Check sheet for the modelled part. Datum: model origin and axes. Units: mm. Round coordinates to 2 decimals unless told otherwise and drop trailing zeros. Order: outer loops, then holes, each group sorted by start corner. A loop starts at its lowest first (then second) coordinate and runs counter-clockwise, first axis right, second up.
Q1. Cross-section at C-C on z = 1.75. Record the cut outline in (x, y).
Q2. Mould release check, pull along X, two halves, no side actions. Record for faces 1 (the flat face through (-31.851, 4, 8)), 2 (the cylindrical face through (28.412, 4.676, 7.736)), 3 (the flat face through (3, 4, 15.341)), 4 (the flat face through (36.149, 4, 8)): +X half, -X half, draft (parallel to the pull), parting line (faces both ways), or undercut.
Q3. Depth check by flat-ended pin: P1, Ø3, axis at x = -13.5, y = 5, coming from the -Z side; P2, Ø1.6, axis at x = 29.15, y = 4, coming from the -Z side. Enter the tip coordinate at first touch or a pass-through.
Q4. Cross-section at A-A on y = 4. Record the cut outline in (x, z), then the cut area to 3 significant figures.
Q5. Cross-section at B-B on x = 29. Record the cut outline in (y, z).
Q6. Scan lines: probe 1 along X at (y, z) = (4, 9.25); probe 2 along Z at (x, y) = (-7, 2); probe 3 along X at (y, z) = (4, 3.75). Record each from-to range of solid material in increasing order.
Q7. Cross-section at D-D on y = 1. Record the cut outline in (x, z), then the cut area to 3 significant figures.
from build123d import *

# Parameters (mm, degrees)
BOSS_EXTRUDE1_DEPTH = 8
SKETCH2_R           = 1
CUT_EXTRUDE1_DEPTH  = 16.340604027


with BuildPart() as part:
    # Sketch1 → Boss-Extrude1 (new body)
    with BuildSketch(Plane(origin=(0, 0, 0), x_dir=(1, 0, 0), z_dir=(0, 1, 0))):
        with BuildLine():
            Line((2.649328859, -0.340604027), (36.149328859, -0.340604027))
            Line((36.149328859, -0.340604027), (36.149328859, -15.340604027))
            Line((36.149328859, -15.340604027), (-31.850671141, -15.340604027))
            Line((-31.850671141, -15.340604027), (-31.850671141, -0.340604027))
            Line((-31.850671141, -0.340604027), (-17.350671141, -0.340604027))
            ThreePointArc((-17.350671141, -0.340604027), (-7.350671141, -10.340604027), (2.649328859, -0.340604027))
        make_face()
    extrude(amount=BOSS_EXTRUDE1_DEPTH)

    # Sketch2 → Cut-Extrude1 (cut, through all)
    with BuildSketch(Plane.XY):
        with Locations((-24.850671141, 4)):
            Circle(SKETCH2_R)
        with Locations((29.149328859, 4)):
            Circle(SKETCH2_R)
    extrude(amount=CUT_EXTRUDE1_DEPTH, mode=Mode.SUBTRACT)


solid = part.part
Results found:
1. outline: (-31.85, 0) - (-17.25, 0) - (-17.25, 8) - (-31.85, 8) - close; (2.55, 0) - (36.15, 0) - (36.15, 8) - (2.55, 8) - close; hole circle Ø2 at (-24.85, 4); hole circle Ø2 at (29.15, 4)
2. face 1: -X half
2. face 2: undercut
2. face 3: draft
2. face 4: +X half
3. P1: stops at z = 6.78
3. P2: passes through
4. outline: (-31.85, 0.34) - (-25.85, 0.34) - (-25.85, 15.34) - (-31.85, 15.34) - close; (-23.85, 0.34) - (-17.35, 0.34) arc R10 cw to (2.65, 0.34) - (28.15, 0.34) - (28.15, 15.34) - (-23.85, 15.34) - close; (30.15, 0.34) - (36.15, 0.34) - (36.15, 15.34) - (30.15, 15.34) - close
4. area: 803 mm2
5. outline: (0, 0.34) - (3.01, 0.34) - (3.01, 15.34) - (0, 15.34) - close; (4.99, 0.34) - (8, 0.34) - (8, 15.34) - (4.99, 15.34) - close
6. probe 1: x = -31.85 to -25.85, -23.85 to -11.89, -2.81 to 28.15, 30.15 to 36.15
6. probe 2: z = 10.33 to 15.34
6. probe 3: x = -31.85 to -25.85, -23.85 to -16.75, 2.05 to 28.15, 30.15 to 36.15
7. outline: (-31.85, 0.34) - (-17.35, 0.34) arc R10 cw to (2.65, 0.34) - (36.15, 0.34) - (36.15, 15.34) - (-31.85, 15.34) - close
7. area: 863 mm2
